Answer from the drawing. Dimensions are ordinates in mm from the lowest x, y and z of the part. A direction names the side the tool comes from. Give positions to 0.01 mm unless a question says otherwise; leave off trailing zeros. Loops run counter-clockwise (first coordinate to the right, second up) from the corner with the lowest first, then second, coordinate; pieces in that order, holes last. Notation, with made-up numbers: (61.25, -19.5) - (88.25, -19.5) arc R20 cw to (88.25, -12.5) - close; hole circle Ø9 at (44.5, 71). An arc over 180 degrees is marked (long way). Write each question's results on one line, items separated by ' | '. Start each with the question number.
Q1. Find the intervals of material crossed by line 1 (Z direction, x = 1.2, y = 3.95); line 2 (Z direction, x = 2.95, y = 3.5); line 3 (Y direction, x = 2.1, z = 11), in increasing order. Write a range as from..to.
Q2. Given pin 1 (1.5 mm diameter, centred on x = 3, z = 5.5, fed in from +Y); pin 2 (0.5 mm diameter, centred on y = 1.5, z = 0.5, fed in from +X), each flat-ended and moving along its own axis, determine where each tip first touches the part or whether it passes through.
Q3. The part is cut by section A-A, the plane x = 2.15. Write down the section's boundary in (y, z) (3 decimals).
Q4. For the marked faces 1 and 2, determine the directions among +Z, -Z, +X, -X, +Y, -Y from which every point of the face is accessible in a straight line to the end or side of a thin tool.
Q5. The part is cut by section C-C, the plane z = 4. Write down the section's boundary in (x, y) (3 decimals).
Q6. The part is cut by section B-B, the plane y = 2.15. Write down the section's boundary in (x, z) (3 decimals).
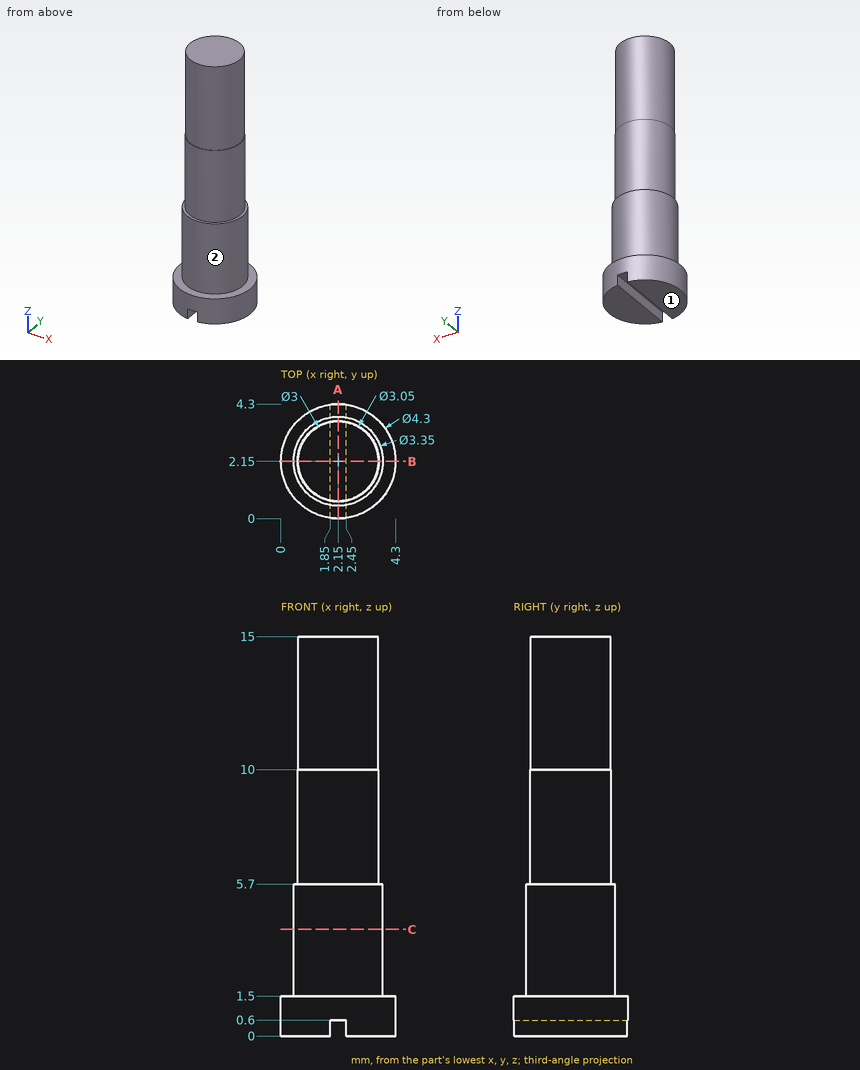
Check sheet entries:
1) line 1: z = 0..1.5 | line 2: z = 0..5.7 | line 3: y = 0.65..3.65
2) pin 1: stops at y = 3.82 | pin 2: stops at x = 4.26
3) outline: (0, 0.6) - (4.3, 0.6) - (4.3, 1.5) - (3.825, 1.5) - (3.825, 5.7) - (3.675, 5.7) - (3.675, 10) - (3.65, 10) - (3.65, 15) - (0.65, 15) - (0.65, 10) - (0.625, 10) - (0.625, 5.7) - (0.475, 5.7) - (0.475, 1.5) - (0, 1.5) - close
4) face 1: -Z, +X, -X, +Y, -Y | face 2: +Z
5) outline: circle Ø3.35 at (2.15, 2.15)
6) outline: (0, 0) - (1.85, 0) - (1.85, 0.6) - (2.45, 0.6) - (2.45, 0) - (4.3, 0) - (4.3, 1.5) - (3.825, 1.5) - (3.825, 5.7) - (3.675, 5.7) - (3.675, 10) - (3.65, 10) - (3.65, 15) - (0.65, 15) - (0.65, 10) - (0.625, 10) - (0.625, 5.7) - (0.475, 5.7) - (0.475, 1.5) - (0, 1.5) - close
